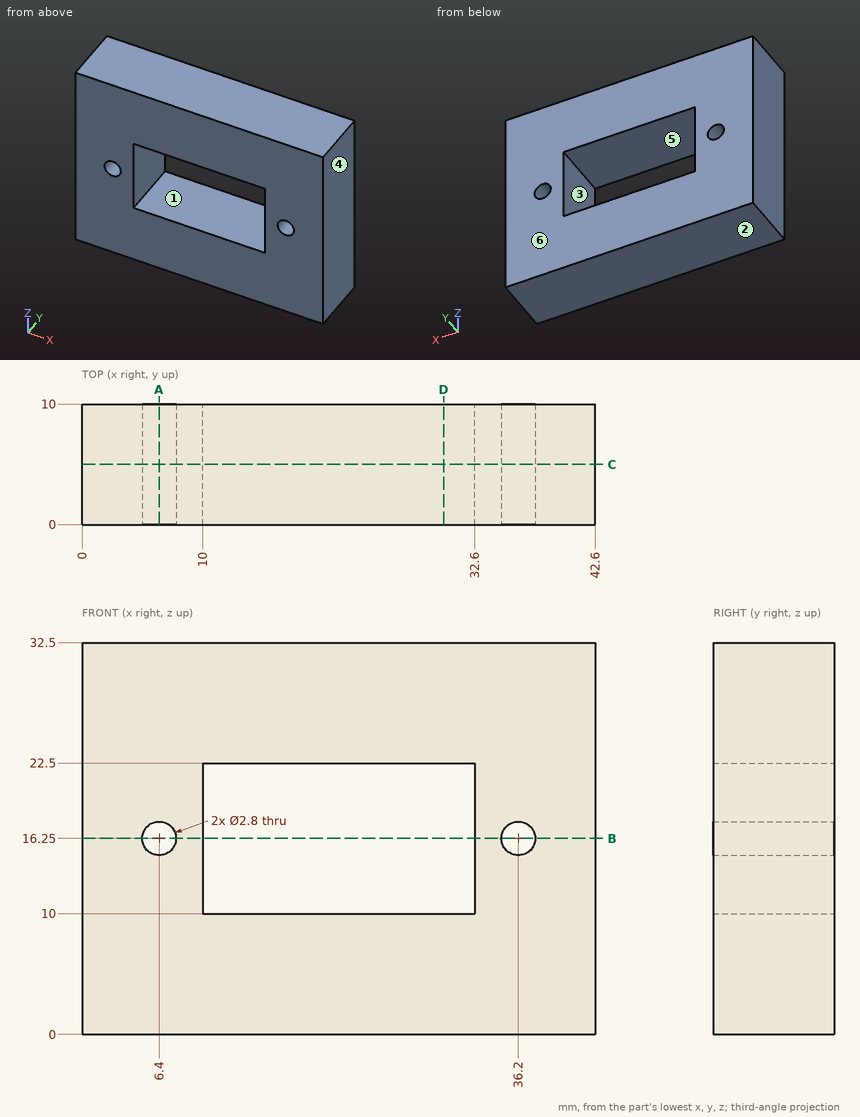
Verification items for this drawing (mm, ordinates from the low corner). A direction names the side the tool comes from. Coordinates: 2 decimals unless noted, no trailing zeros. Loops run counter-clockwise (first coordinate to the right, second up) from the corner with the lowest first, then second, coordinate; pieces in that order, holes last.
Item 1: Release check for a two-part mould opening along X. For the marked faces 1, 2, 3 and 4 record: released by +X, released by -X, zero draft, split by the parting line, or undercut.
Item 2: Sectioned sample at A-A, the plane x = 6.4. Record the boundary of the cut face in (y, z).
Item 3: Thickness scan on line 1 (X direction, y = 8, z = 16.25); line 2 (Z direction, x = 36.2, y = 6); line 3 (X direction, y = 3.25, z = 11). Record the ranges inside material, lowest first.
Item 4: Access from +Z, -Z, +X, -X, +Y, -Y to the whole of each face (thin tool, end or side, straight path). Record for the marked faces 5 and 6.
Item 5: Go/stop test with a flat-tipped pin: pin 1 Ø3 at (x, z) = (6.4, 16.25) entering from -Y. Record where the tip stops, or that it passes through.
Item 6: Sectioned sample at D-D, the plane x = 30. Record the boundary of the cut face in (y, z).
Item 7: Sectioned sample at C-C, the plane y = 5. Record the boundary of the cut face in (x, z), then the cut area to 3 significant figures.
Item 8: Sectioned sample at B-B, the plane z = 16.25. Record the boundary of the cut face in (x, y), then the cut area to 3 significant figures.
Check result:
1. face 1: undercut
1. face 2: zero draft
1. face 3: undercut
1. face 4: released by +X
2. outline: (0, 0) - (10, 0) - (10, 14.85) - (0, 14.85) - close; (0, 17.65) - (10, 17.65) - (10, 32.5) - (0, 32.5) - close
3. line 1: x = 0 to 5, 7.8 to 10, 32.6 to 34.8, 37.6 to 42.6
3. line 2: z = 0 to 14.85, 17.65 to 32.5
3. line 3: x = 0 to 10, 32.6 to 42.6
4. face 5: +Y, -Y
4. face 6: +Z, -Z, +X, -X, +Y
5. pin 1: stops at y = 0
6. outline: (0, 0) - (10, 0) - (10, 10) - (0, 10) - close; (0, 22.5) - (10, 22.5) - (10, 32.5) - (0, 32.5) - close
7. outline: (0, 0) - (42.6, 0) - (42.6, 32.5) - (0, 32.5) - close; hole circle Ø2.8 at (6.4, 16.25); hole (10, 10) - (32.6, 10) - (32.6, 22.5) - (10, 22.5) - close; hole circle Ø2.8 at (36.2, 16.25)
7. area: 1,090 mm2
8. outline: (0, 0) - (5, 0) - (5, 10) - (0, 10) - close; (7.8, 0) - (10, 0) - (10, 10) - (7.8, 10) - close; (32.6, 0) - (34.8, 0) - (34.8, 10) - (32.6, 10) - close; (37.6, 0) - (42.6, 0) - (42.6, 10) - (37.6, 10) - close
8. area: 144 mm2
